Here's how the part is built. I have some questions about the finished solid (model axes, mm). Round coordinates to 2 decimals unless told otherwise and drop trailing zeros. Order: outer loops, then holes, each group sorted by start corner. A loop starts at its lowest first (then second) coordinate and runs counter-clockwise, first axis right, second up. Notation, with made-up numbers: (55.25, 84) -> (81.25, 84) arc R26 ccw to (81.25, 123) -> close; hole circle Ø5 at (1.25, -22.5). An arc over 180 degrees is marked (long way). Answer in a Markdown table with one row per item.
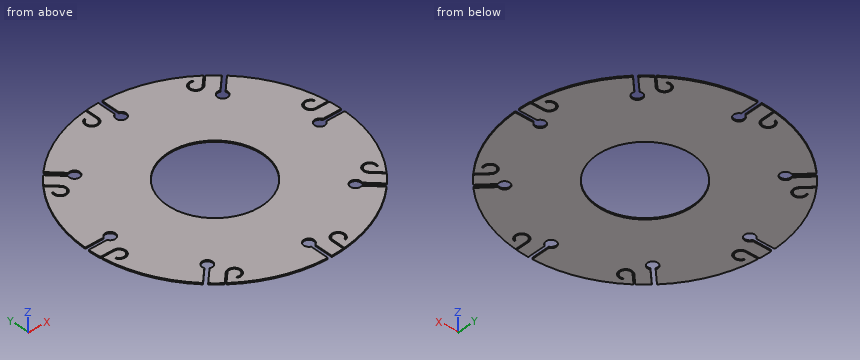
```python
from build123d import *

# Parameters (mm, degrees)
F0_R            = 185
F2_DEPTH        = 5
F3_DEPTH        = 5
F3_COPIES_COUNT = 8
F4_R            = 2


# Not quite as in the source:
# - a pattern or mirror of a feature is missing from the dataset's text; its kind, count and spacing are read off the source's solid
# - a feature names something its author has since deleted; it is built from what else it names


with BuildPart() as f2:
    # F0 (on Top) → F2 (new body)
    with BuildSketch(Plane.XY):
        with BuildLine():
            ThreePointArc((-491.3501806248, -60), (30.055453671, -494.0867026187), (495, 0))
            ThreePointArc((495, 0), (3.750107621, 494.9857944354), (-494.9431785569, 7.5))
            Line((-494.9431785569, 7.5), (-424.843134833, 7.5))
            ThreePointArc((-424.843134833, 7.5), (-423.7771312512, 7.8077717755), (-423.0392134845, 8.6363636364))
            ThreePointArc((-423.0392134845, 8.6363636364), (-385, 0), (-423.0392134845, -8.6363636364))
            ThreePointArc((-423.0392134845, -8.6363636364), (-423.7771312512, -7.8077717755), (-424.843134833, -7.5))
            Line((-424.843134833, -7.5), (-494.9431785569, -7.5))
            ThreePointArc((-494.9431785569, -7.5), (-494.0102986253, -31.2861766946), (-491.93495505, -55))
            Line((-491.93495505, -55), (-441.93495505, -55))
            ThreePointArc((-441.93495505, -55), (-420.5886816099, -93.0129401067), (-464.1571772722, -91.4530711823))
            ThreePointArc((-464.1571772722, -91.4530711823), (-463.0802621682, -88.0855418418), (-459.7127328277, -89.1624569458))
            ThreePointArc((-459.7127328277, -89.1624569458), (-424.8579362979, -90.4103520854), (-441.93495505, -60))
            Line((-441.93495505, -60), (-491.3501806248, -60))
        make_face()
        Circle(F0_R, mode=Mode.SUBTRACT)
        with BuildLine():
            Line((-424.843134833, 7.5), (-494.9431785569, 7.5))
            ThreePointArc((-494.9431785569, 7.5), (-495, 0), (-494.9431785569, -7.5))
            Line((-494.9431785569, -7.5), (-424.843134833, -7.5))
            ThreePointArc((-424.843134833, -7.5), (-423.7771312512, -7.8077717755), (-423.0392134845, -8.6363636364))
            ThreePointArc((-423.0392134845, -8.6363636364), (-385, 0), (-423.0392134845, 8.6363636364))
            ThreePointArc((-423.0392134845, 8.6363636364), (-423.7771312512, 7.8077717755), (-424.843134833, 7.5))
        make_face()
        with BuildLine():
            ThreePointArc((-491.93495505, -55), (-491.64892404, -57.500743389), (-491.3501806248, -60))
            Line((-491.3501806248, -60), (-441.93495505, -60))
            ThreePointArc((-441.93495505, -60), (-424.8579362979, -90.4103520854), (-459.7127328277, -89.1624569458))
            ThreePointArc((-459.7127328277, -89.1624569458), (-463.0802621682, -88.0855418418), (-464.1571772722, -91.4530711823))
            ThreePointArc((-464.1571772722, -91.4530711823), (-420.5886816099, -93.0129401067), (-441.93495505, -55))
            Line((-441.93495505, -55), (-491.93495505, -55))
        make_face()
    extrude(amount=F2_DEPTH)

    # F0 (on Top) → F3 (cut, through all)
    with BuildSketch(Plane.XY):
        with BuildLine():
            Line((-424.843134833, 7.5), (-494.9431785569, 7.5))
            ThreePointArc((-494.9431785569, 7.5), (-495, 0), (-494.9431785569, -7.5))
            Line((-494.9431785569, -7.5), (-424.843134833, -7.5))
            ThreePointArc((-424.843134833, -7.5), (-423.7771312512, -7.8077717755), (-423.0392134845, -8.6363636364))
            ThreePointArc((-423.0392134845, -8.6363636364), (-385, 0), (-423.0392134845, 8.6363636364))
            ThreePointArc((-423.0392134845, 8.6363636364), (-423.7771312512, 7.8077717755), (-424.843134833, 7.5))
        make_face()
        with BuildLine():
            ThreePointArc((-491.93495505, -55), (-491.64892404, -57.500743389), (-491.3501806248, -60))
            Line((-491.3501806248, -60), (-441.93495505, -60))
            ThreePointArc((-441.93495505, -60), (-424.8579362979, -90.4103520854), (-459.7127328277, -89.1624569458))
            ThreePointArc((-459.7127328277, -89.1624569458), (-463.0802621682, -88.0855418418), (-464.1571772722, -91.4530711823))
            ThreePointArc((-464.1571772722, -91.4530711823), (-420.5886816099, -93.0129401067), (-441.93495505, -55))
            Line((-441.93495505, -55), (-491.93495505, -55))
        make_face()
    f3 = extrude(amount=F3_DEPTH, mode=Mode.SUBTRACT)

    # F3_copies: F3 ×8 about axis
    f3_copies_axis = Axis((0, 0, 0), (0, 0, 1))
    for i in range(1, F3_COPIES_COUNT):
        add(f3.rotate(f3_copies_axis, i * 360 / F3_COPIES_COUNT), mode=Mode.SUBTRACT)

    # F4
    f4_edges = [f2.edges().sort_by_distance(p)[0] for p in [
        (-494.943179, -7.5, 2.5),
        (-494.943179, 7.5, 2.5),
        (-491.934955, -55, 2.5),
        (-491.350181, -60, 2.5),
        (-355.280979, -344.674377, 2.5),
        (-389.863452, 305.010638, 2.5),
        (-386.741416, 308.95967, 2.5),
        (-355.280979, 344.674377, 2.5),
        (-344.674377, 355.280979, 2.5),
        (-60, 491.350181, 2.5),
        (-55, 491.934955, 2.5),
        (-7.5, 494.943179, 2.5),
        (7.5, 494.943179, 2.5),
        (305.010638, 389.863452, 2.5),
        (308.95967, 386.741416, 2.5),
        (344.674377, 355.280979, 2.5),
        (355.280979, 344.674377, 2.5),
        (491.350181, 60, 2.5),
        (491.934955, 55, 2.5),
        (494.943179, 7.5, 2.5),
        (494.943179, -7.5, 2.5),
        (389.863452, -305.010638, 2.5),
        (386.741416, -308.95967, 2.5),
        (355.280979, -344.674377, 2.5),
        (344.674377, -355.280979, 2.5),
        (60, -491.350181, 2.5),
        (55, -491.934955, 2.5),
        (7.5, -494.943179, 2.5),
        (-7.5, -494.943179, 2.5),
        (-305.010638, -389.863452, 2.5),
        (-308.95967, -386.741416, 2.5),
        (-344.674377, -355.280979, 2.5),
    ]]
    fillet(f4_edges, radius=F4_R)


solid = f2.part
```
1. Please list where these lines run through material, in increasing order: line 1 along X through (y, z) = (334, 1.4); line 2 along X through (y, z) = (-95, 4.55); line 3 along Y through (x, z) = (-80, 1.55).
Numbers:
| item | result |
|---|---|
| line 1 | x = -365.33 to -344.61, -323.39 to 323.39, 344.61 to 365.33 |
| line 2 | x = -485.8 to -461.93, -455.16 to -428.71, -421.93 to -158.75, 158.75 to 485.8 |
| line 3 | y = -488.49 to -166.81, 166.81 to 416.93, 421.93 to 488.49 |
2. For pin 1 Ø3 at (x, z) = (108, 2) entering from +Y; pin 2 Ø1 at (y, z) = (-65.5, 3) entering from -X; pin 3 Ø2.5 at (x, z) = (-442.5, 2) entering from -Y, each with a flat end and sliding along its axis, tell me the tip position at first contact or that it passes through.
Numbers:
| item | result |
|---|---|
| pin 1 | stops at y = 483.41 |
| pin 2 | stops at x = -490.71 |
| pin 3 | stops at y = -224.33 |
3. Suppose I cut it at B-B on x = -152.5. Write out the boundary of the cut face in (y, z).
Numbers:
| item | result |
|---|---|
| outline | (-470.92, 0) -> (-104.73, 0) -> (-104.73, 5) -> (-470.92, 5) -> close; (104.73, 0) -> (470.92, 0) -> (470.92, 5) -> (104.73, 5) -> close |
4. Suppose I cut it at A-A on y = -371. Write out the boundary of the cut face in (x, z).
Numbers:
| item | result |
|---|---|
| outline | (-327.69, 0) -> (-293.22, 0) -> (-293.22, 5) -> (-327.69, 5) -> close; (-286.15, 0) -> (-236.02, 0) -> (-236.02, 5) -> (-286.15, 5) -> close; (-231, 0) -> (327.69, 0) -> (327.69, 5) -> (-231, 5) -> close |
